The listing builds one solid part. Answer for the finished solid, in the listing's coordinates (mm). Give positions to 0.01 mm unless a question says otherwise; leave off trailing zeros. Write each loop counter-clockwise with the first axis right and the second up, starting at its lowest first coordinate (ties: lowest second). Pieces come first, ordered by that corner, then holes. Notation, with made-up numbers: (-6, 42.5) -> (2, 42.5) arc R28 cw to (2, 71.5) -> close; hole circle Ø5 at (-21.5, -38.5). An arc over 180 degrees is marked (long way). Write each question's results on one line, items separated by ' | '. Start each with the question number.
from build123d import *

# Parameters (mm, degrees)
SKETCH1_W           = 20
SKETCH1_H           = 400
BOSS_EXTRUDE1_DEPTH = 10
FILLET1_R           = 10
SKETCH2_R           = 5
CUT_EXTRUDE1_DEPTH  = 201.499376558
SKETCH3_R           = 5
BOSS_EXTRUDE2_DEPTH = 20
FILLET2_R           = 5


with BuildPart() as part:
    # Sketch1 → Boss-Extrude1 (new body)
    with BuildSketch(Plane.XY):
        Rectangle(SKETCH1_W, SKETCH1_H)
    extrude(amount=BOSS_EXTRUDE1_DEPTH)

    # Fillet1
    fillet1_edges = [part.edges().sort_by_distance(p)[0] for p in [
        (-10, -200, 5),
        (10, -200, 5),
        (-10, 200, 5),
        (10, 200, 5),
    ]]
    fillet(fillet1_edges, radius=FILLET1_R - 0.0001)  # a hair under: the kernel refuses the full size

    # Sketch2 → Cut-Extrude1 (cut, through all)
    with BuildSketch(Plane.XY.offset(10)):
        with Locations((0, 191.5)):
            Circle(SKETCH2_R)
    cut_extrude1 = extrude(amount=-CUT_EXTRUDE1_DEPTH, mode=Mode.SUBTRACT)

    # Mirror1: Cut-Extrude1 across plane
    add(cut_extrude1.mirror(Plane.ZX), mode=Mode.SUBTRACT)

    # Sketch3 → Boss-Extrude2 (add)
    with BuildSketch(Plane(origin=(0, 0, 0), x_dir=(-1, 0, 0), z_dir=(0, 0, -1))):
        with Locations((0, 161.5)):
            Circle(SKETCH3_R)
    extrude(amount=BOSS_EXTRUDE2_DEPTH)

    # Fillet2
    fillet2_edges = [part.edges().sort_by_distance(p)[0] for p in [
        (5, 161.5, 0),
    ]]
    fillet(fillet2_edges, radius=FILLET2_R - 0.0001)  # a hair under: the kernel refuses the full size


solid = part.part
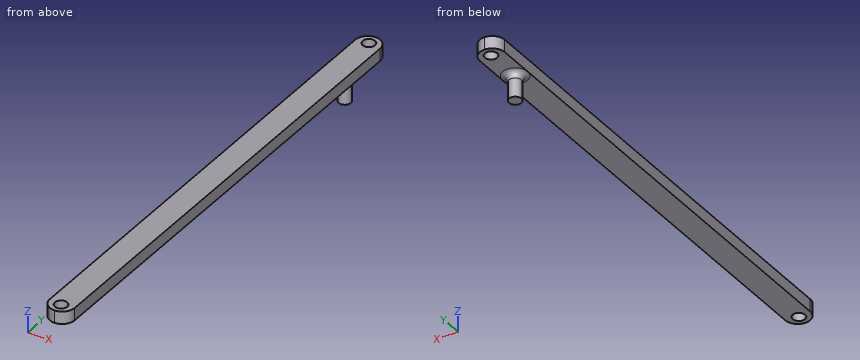
1. Each of these flat-tipped pins is pushed along its axis until it touches: pin 1 Ø6 at (x, z) = (7, -12.5) entering from -Y; pin 2 Ø6 at (x, z) = (-4.5, 2) entering from -Y; pin 3 Ø10 at (x, y) = (4.5, -97) entering from -Z. Where does it stop, or does it pass through?
2. Consider probe 1 along Y at (x, z) = (0, 7); probe 2 along Y at (x, z) = (1.25, 6.75); probe 3 along Z at (x, y) = (-3.75, -82). Determine where each line is inside the solid, lowest interval first. Write a range as [from, to].
3. Section C-C (y = 23) is taken. Write down the section's boundary in (x, z).
4. Section A-A (z = 3.75) is taken. Give the number of separate pieces and of enclosed holes in the cut face, then the cut area to 3 significant figures.
Results:
1) pin 1: stops at y = 158.5 | pin 2: stops at y = -199.89 | pin 3: stops at z = 0
2) probe 1: y = [-200, -196.5], [-186.5, 186.5], [196.5, 200] | probe 2: y = [-199.92, -196.34], [-186.66, 186.66], [196.34, 199.92] | probe 3: z = [0, 10]
3) outline: (-10, 0) -> (10, 0) -> (10, 10) -> (-10, 10) -> close
4) separate pieces: 1 | enclosed holes: 2 | area: 7,760 mm²
